Solid Edge part; units mm, degrees
sketch "Sketch1" plane through (0, 0, 0) normal (0, 0, 1) x (1, 0, 0)
  arc A0 (0, -4) -> (0, 4) centre (0, 0) cw
  line L0 (0, 4) -> (6, 4)
  line L1 (6, 4) -> (6, 2)
  line L2 (6, 2) -> (29, 2)
  line L3 (29, 2) -> (29, 3)
  line L4 (35, 3) -> (29, 3)
  arc A1 (35, 3) -> (35, -3) centre (35, 0) cw
  line L5 (35, -3) -> (29, -3)
  line L6 (29, -2) -> (29, -3)
  line L7 (6, -2) -> (29, -2)
  line L8 (6, -4) -> (6, -2)
  line L9 (0, -4) -> (6, -4)
extrude "Protrusion1" add sketch "Sketch1" along normal blind 3
sketch "Sketch2" plane through (17, 0, 3) normal (0, 0, 1) x (1, 0, 0)
  circle A0 centre (-17, 0) radius 2
  circle A1 centre (18, 0) radius 1.5
extrude "Cutout1" cut sketch "Sketch2" against normal through all
fillet "Rounding" radius 8 4 edges at (6, -2, 1.5) (6, 2, 1.5) (29, 2, 1.5) (29, -2, 1.5)
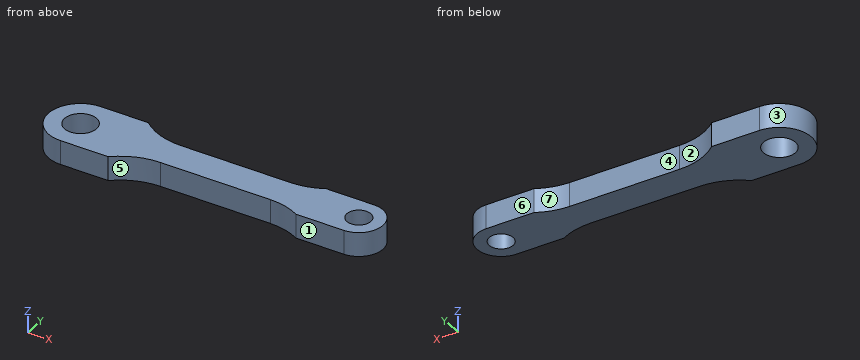
Design review of the part built by this model. Coordinates are the model's own, in mm. Face numbers are marked on the shaded views. A direction names the side the tool comes from. Round coordinates to 2 decimals unless told otherwise and drop trailing zeros. Write each loop counter-clockwise with the first axis right and the second up, starting at its lowest first coordinate (ties: lowest second). Pieces come first, ordered by that corner, then holes. Notation, with made-up numbers: (-33, 49) -> (-18, 49) arc R20 ccw to (-18, 81) -> close; hole circle Ø5 at (40, 51). An arc over 180 degrees is marked (long way). Answer in a Markdown table with one row per item.
Q1. Clearance check with flat-ended pins moving along their axes: pin 1 Ø0.9 at (x, z) = (21.5, 2) entering from +Y; pin 2 Ø0.9 at (x, z) = (31.5, 2) entering from -Y. State where each tip first meets the part, or that it passes through.
The answers:
| item | result |
|---|---|
| pin 1 | y = 2 |
| pin 2 | y = -3 |
Q2. For the marked faces 5, 6 and 7, list the 3-axis set-ups (+Z, -Z, +X, -X, +Y, -Y) from which the entire face can be reached by the end or side of a thin tool; tool diameter is ignored.
The answers:
| item | result |
|---|---|
| face 5 | +Z, -Z, -Y |
| face 6 | +Z, -Z, +X, +Y |
| face 7 | +Z, -Z, +Y |
Q3. Take a section at A-A, the plane z = 1.5. State the section outline as (x, y) points, then the cut area to 3 significant figures.
The answers:
| item | result |
|---|---|
| outline | (0, -4) -> (6, -4) arc R8 cw to (11.29, -2) -> (25.13, -2) arc R8 cw to (29, -3) -> (35, -3) arc R3 ccw to (35, 3) -> (29, 3) arc R8 cw to (25.13, 2) -> (11.29, 2) arc R8 cw to (6, 4) -> (0, 4) arc R4 ccw to start; hole circle Ø4 at (0, 0); hole circle Ø3 at (35, 0) |
| area | 205 mm² |
Q4. Draft analysis for pull direction X (two halves, no side actions). For the marked faces 1, 2, 3 and 4, state which applies: +X half, -X half, draft (parallel to the pull), parting line (faces both ways), or undercut.
The answers:
| item | result |
|---|---|
| face 1 | draft |
| face 2 | undercut |
| face 3 | -X half |
| face 4 | undercut |
Q5. Take a section at B-B, the plane x = 22.5. State the section outline as (y, z) points, then the cut area to 3 significant figures.
The answers:
| item | result |
|---|---|
| outline | (-2, 0) -> (2, 0) -> (2, 3) -> (-2, 3) -> close |
| area | 12.0 mm² |
Q6. To check wall thickness, follow L1, parallel to Y at x = 35, z = 1; L2, parallel to Y at x = 0, z = 1.05; L3, parallel to X at y = 0.5, z = 0.2. State the ranges of each line that lie inside material, in increasing order. Write a range as [from, to].
The answers:
| item | result |
|---|---|
| L1 | [-3, -1.5], [1.5, 3] |
| L2 | [-4, -2], [2, 4] |
| L3 | [-3.97, -1.94], [1.94, 33.59], [36.41, 37.96] |
